```python
from build123d import *

# Parameters (mm, degrees)
F0_W     = 508
F0_H     = 508
F2_DEPTH = 6.35
F3_W     = 469.9
F3_H     = 79.375
F4_DEPTH = 76.2


with BuildPart() as f2:
    # F0 (on Front) → F2 (new body)
    with BuildSketch(Plane.XZ):
        with Locations((254, 254)):
            Rectangle(F0_W, F0_H)
    extrude(amount=F2_DEPTH)

    # F3 (on face) → F4 (join)
    with BuildSketch(Plane.XZ.offset(6.35)):
        Polygon((0, 508), (0, 0), (19.05, 0), (19.05, 428.625), (19.05, 508), align=None)
        with Locations((254, 468.3125)):
            Rectangle(F3_W, F3_H)
        Polygon((488.95, 508), (488.95, 428.625), (488.95, 0), (508, 0), (508, 508), align=None)
    extrude(amount=F4_DEPTH)


solid = f2.part
```
Source: CAD feature listing. Evaluate the final solid. Frame: model axes, mm. A direction names the side the tool comes from. Round coordinates to 2 decimals unless told otherwise and drop trailing zeros. Loops run counter-clockwise (first coordinate to the right, second up) from the corner with the lowest first, then second, coordinate; pieces in that order, holes last. Notation, with made-up numbers: M 58,17 L 116,17 A17 ccw 116,46 Z; hole C -28,76.5 d7. An arc over 180 degrees is marked long. Use a Markdown table: item, result. Add a question column.
1. Cut plane B-B, the plane y = -30. Output: boundary loops of the cut face in (x, z) (3 decimals), and give its area (3 significant figures).
2. Cut plane A-A, the plane z = 407. Output: boundary loops of the cut face in (x, y), and give its area (3 significant figures).
3. Cut plane C-C, the plane x = 325.5. Output: boundary loops of the cut face in (y, z) (3 decimals).
4. Ray query, line 1 along X through (y, z) = (-14, 89); line 2 along Z through (x, y) = (368, -8.5) (3 decimals). Return the intervals inside material, ascending. Write a range as [from, to].
5. Contact query for flat-ended pins moving along their axis: pin 1 (8 mm diameter, centred on y = -10.5, z = 301.5, fed in from -X); pin 2 (1 mm diameter, centred on x = 456, z = 410.5, fed in from -Y); pin 3 (3 mm diameter, centred on x = 298, y = -13.5, fed in from -Z) (3 decimals). Output: stop coordinate, or through.
6. Set-up query: faces 1 (the flat face through (251, -44, 428.625)), 2 (the flat face through (0, -41, 258)). Return all of +Z, -Z, +X, -X, +Y, -Y with unobstructed straight access to the full face (end or side cutting, diameter ignored); none if empty.
7. Pull-direction query (X, two-part tool) for faces 3 (the flat face through (253, -1, 0)), 4 (the flat face through (251, -6.35, 217)), 5 (the flat face through (508, -41, 250)); classes: +X half, -X half, draft (parallel to the pull), parting line (faces both ways), or undercut.
Solution:
| question | item | result |
|---|---|---|
| 1 | outline | M 0,0 L 19.05,0 L 19.05,428.625 L 488.95,428.625 L 488.95,0 L 508,0 L 508,508 L 0,508 Z |
| 1 | area | 56,700 mm2 |
| 2 | outline | M 0,-82.55 L 19.05,-82.55 L 19.05,-6.35 L 488.95,-6.35 L 488.95,-82.55 L 508,-82.55 L 508,0 L 0,0 Z |
| 2 | area | 6,130 mm2 |
| 3 | outline | M -82.55,428.625 L -6.35,428.625 L -6.35,0 L 0,0 L 0,508 L -82.55,508 Z |
| 4 | line 1 | x = [0, 19.05], [488.95, 508] |
| 4 | line 2 | z = [428.625, 508] |
| 5 | pin 1 | stops at x = 0 |
| 5 | pin 2 | stops at y = -6.35 |
| 5 | pin 3 | stops at z = 428.625 |
| 6 | face 1 | -Z, -Y |
| 6 | face 2 | +Z, -Z, -X, +Y, -Y |
| 7 | face 3 | draft |
| 7 | face 4 | undercut |
| 7 | face 5 | +X half |
